Part print with two shaded views. Sizes in mm from the minimum x, y, z corner. Give positions to 0.01 mm unless a question says otherwise; leave off trailing zeros. Order: outer loops, then holes, each group sorted by start corner. A loop starts at its lowest first (then second) coordinate and runs counter-clockwise, first axis right, second up. Notation, with made-up numbers: (3.25, 27.25) - (30.25, 27.25) arc R24 ccw to (30.25, 66.25) - close; hole circle Ø8 at (-10, 12). An arc over 180 degrees is marked (long way). Return JSON: item names as keys, results as strings. Group by question number.
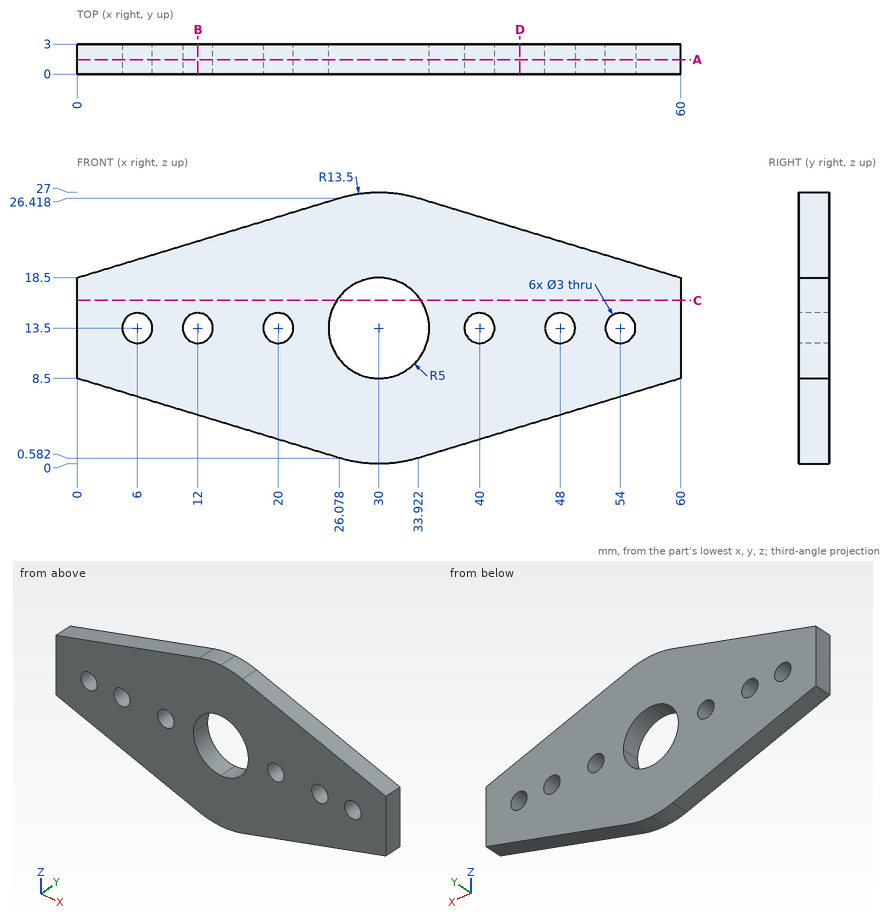
(1) Slice it at B-B (x = 12). Give the cut face in (y, z).
(2) Drill centre lines: L1, parallel to Z at x = 20, y = 2.8; L2, parallel to Z at x = 54.5, y = 0.4 (1 decimal); L3, parallel to X at y = 1.8, z = 18. Where is each one in solid material? Low to high.
(3) Slice it at D-D (x = 44). Give the cut face in (y, z).
(4) Slice it at A-A (y = 1.45). Give the cut face in (x, z).
(5) Slice it at C-C (z = 16.25). Give the cut face in (x, y), and give its area (3 significant figures).
Result set:
{
 "1": {"outline": "(0, 4.86) - (3, 4.86) - (3, 12) - (0, 12) - close; (0, 15) - (3, 15) - (3, 22.14) - (0, 22.14) - close"},
 "2": {"L1": "z = 2.43 to 12, 15 to 24.57", "L2": "z = 6.8 to 12.1, 14.9 to 20.2", "L3": "x = 0 to 27.82, 32.18 to 60"},
 "3": {"outline": "(0, 3.64) - (3, 3.64) - (3, 23.36) - (0, 23.36) - close"},
 "4": {"outline": "(0, 8.5) - (26.08, 0.58) arc R13.5 ccw to (33.92, 0.58) - (60, 8.5) - (60, 18.5) - (33.92, 26.42) arc R13.5 ccw to (26.08, 26.42) - (0, 18.5) - close; hole circle Ø3 at (6, 13.5); hole circle Ø3 at (12, 13.5); hole circle Ø3 at (20, 13.5); hole circle Ø10 at (30, 13.5); hole circle Ø3 at (40, 13.5); hole circle Ø3 at (48, 13.5); hole circle Ø3 at (54, 13.5)"},
 "5": {"outline": "(0, 0) - (25.82, 0) - (25.82, 3) - (0, 3) - close; (34.18, 0) - (60, 0) - (60, 3) - (34.18, 3) - close", "area": "155 mm²"}
}
